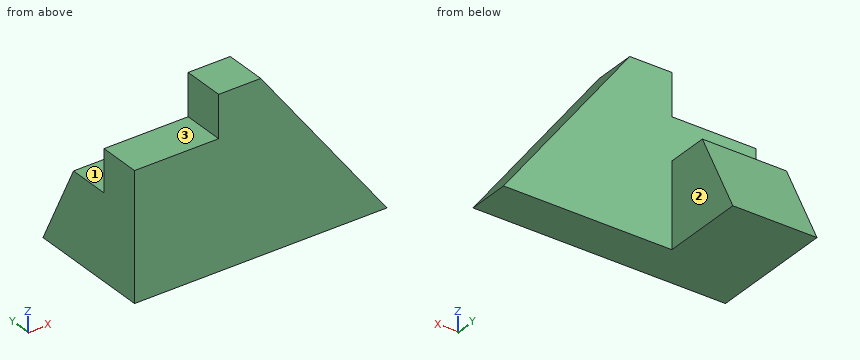
```python
from build123d import *

# Parameters (mm, degrees)
EXTRUDE_1_DEPTH = 5
EXTRUDE_2_DEPTH = 10


with BuildPart() as part:
    # 草圖1 → 填料-伸長1 (new body)
    with BuildSketch(Plane(origin=(0, 0, 0), x_dir=(1, 0, 0), z_dir=(0, 1, 0))):
        Polygon((0, 0), (30, 0), (15, -20), (10, -20), (10, -15), (0, -15), align=None)
    extrude(amount=EXTRUDE_1_DEPTH)

    # 草圖2 → 填料-伸長2 (add)
    with BuildSketch(Plane.ZY):
        Polygon((0, 5), (0, 15), (10, 10), (10, 5), align=None)
    extrude(amount=-EXTRUDE_2_DEPTH)


solid = part.part
```
Work out the finished part from the listing and answer in its coordinate system (mm). Face numbers are marked on the shaded views. A direction names the side the tool comes from. Round coordinates to 2 decimals unless told otherwise and drop trailing zeros. Order: outer loops, then holes, each group sorted by start corner. A loop starts at its lowest first (then second) coordinate and runs counter-clockwise, first axis right, second up.
Q1. A cutting plane is placed at D-D, the plane x = 13.75. Determine the outline of the cut face in (y, z).
Solution:
outline: (0, 0) - (5, 0) - (5, 20) - (0, 20) - close
Q2. Given pin 1 Ø1.5 at (x, y) = (9.5, 10.5) entering from +Z; pin 2 Ø4 at (x, y) = (2.5, 6.5) entering from +Z; pin 3 Ø4 at (x, z) = (9, 3.5) entering from +Y, each flat-ended and moving along its own axis, determine where each tip first touches the part or whether it passes through.
Solution:
pin 1: stops at z = 10
pin 2: stops at z = 15
pin 3: stops at y = 14.25
Q3. A tool of negligible diameter and unlimited length cuts with its end or side. For the marked faces 1, 2 and 3, from which of +Z, -Z, +X, -X, +Y, -Y can it reach the whole face along a straight path? Write none if from no direction.
Solution:
face 1: +Z, +X, -X, +Y
face 2: +Z, -Z, +X, +Y
face 3: +Z, -X, +Y, -Y
Q4. A cutting plane is placed at B-B, the plane x = 5.25. Determine the outline of the cut face in (y, z), then the cut area to 3 significant figures.
Solution:
outline: (0, 0) - (15, 0) - (10, 10) - (5, 10) - (5, 15) - (0, 15) - close
area: 150 mm2
Q5. Find the intervals of material crossed by line 1 along X through (y, z) = (9.5, 3.25); line 2 along Y through (x, z) = (14, 6.75), in increasing order.
Solution:
line 1: x = 0 to 10
line 2: y = 0 to 5
Q6. A cutting plane is placed at A-A, the plane z = 6. Determine the outline of the cut face in (x, y).
Solution:
outline: (0, 0) - (25.5, 0) - (25.5, 5) - (10, 5) - (10, 12) - (0, 12) - close
Q7. A cutting plane is placed at C-C, the plane y = 11.5. Determine the outline of the cut face in (x, z).
Solution:
outline: (0, 0) - (10, 0) - (10, 7) - (0, 7) - close
